from build123d import *

# Parameters (mm, degrees)
BASPROSKE_W         = 5
BASPROSKE_H         = 19
TOOTHCUT_DEPTH      = 28.331300737
TEETHCUTS_COUNT     = 17
BORSKE_R            = 4
BORE_DEPTH          = 50.0000508
BOSS_EXTRUDE1_DEPTH = 5


with BuildPart() as part:
    # BasProSke → Base-Revolve (revolve)
    with BuildSketch(Plane(origin=(0, 0, 0), x_dir=(1, 0, 0), z_dir=(0, 1, 0)), mode=Mode.PRIVATE) as base_revolve_sk:
        with Locations((2.5, 9.5)):
            Rectangle(BASPROSKE_W, BASPROSKE_H)
    revolve(base_revolve_sk.sketch.rotate(Axis((-10, 0, 0), (1, 0, 0)), 180), axis=Axis((-10, 0, 0), (1, 0, 0)))

    # TooCutSke → ToothCut (cut, through all)
    with BuildSketch(Plane(origin=(0, 0, 0), x_dir=(0, 0, -1), z_dir=(1, 0, 0))):
        with BuildLine():
            ThreePointArc((1.020352389, 14.463052306), (0, 14.499), (-1.020352389, 14.463052306))
            ThreePointArc((-1.020352389, 14.463052306), (-1.632621885, 16.804485203), (-3.026143023, 18.783192049))
            ThreePointArc((-3.026143023, 18.783192049), (0, 19.0254), (3.026143023, 18.783192049))
            ThreePointArc((3.026143023, 18.783192049), (1.632621885, 16.804485203), (1.020352389, 14.463052306))
        make_face()
    toothcut = extrude(amount=TOOTHCUT_DEPTH, mode=Mode.SUBTRACT)

    # TeethCuts: ToothCut ×17 about axis
    teethcuts_axis = Axis((0, 0, 0), (1, 0, 0))
    for i in range(1, TEETHCUTS_COUNT):
        add(toothcut.rotate(teethcuts_axis, i * 360 / TEETHCUTS_COUNT), mode=Mode.SUBTRACT)

    # BorSke → Bore (cut, symmetric)
    with BuildSketch(Plane(origin=(0, 0, 0), x_dir=(0, 0, -1), z_dir=(1, 0, 0))):
        with Locations(Location((0, 0, 0), (0, 0, 180))):
            Circle(BORSKE_R)
    extrude(amount=BORE_DEPTH, both=True, mode=Mode.SUBTRACT)

    # Sketch1 → Boss-Extrude1 (add)
    with BuildSketch(Plane(origin=(5, 0, 0), x_dir=(0, 0, -1), z_dir=(1, 0, 0))):
        with BuildLine():
            ThreePointArc((3.122498999, 2.5), (0, 4), (-3.122498999, 2.5))
            Line((-3.122498999, 2.5), (3.122498999, 2.5))
        make_face()
    extrude(amount=-BOSS_EXTRUDE1_DEPTH)


solid = part.part
Could you check a few things on this model? Use its own coordinates, in mm. A direction names the side the tool comes from. Coordinates: 2 decimals unless noted, no trailing zeros. Loops run counter-clockwise (first coordinate to the right, second up) from the corner with the lowest first, then second, coordinate; pieces in that order, holes last.
1. For faces 1 (the face through (3, 2.5, 0)), 2 (the face through (2.465, -11.386, 12.403)), 3 (the face through (2.46, 11.3, 12.48)), which set-ups out of +Z, -Z, +X, -X, +Y, -Y let a thin tool reach every point of the face, with its end or its side?
2. For P1, Ø2, axis at y = -8.5, z = -4.5, coming from the -X side; P2, Ø1.5, axis at x = 2, z = -8, coming from the -Y side; P3, Ø2, axis at x = 1, y = 6, coming from the -Z side; P4, Ø2, axis at x = 4.5, z = -4.5, coming from the -Y side, each with a flat end and sliding along its axis, tell me the tip position at first contact or that it passes through.
3. We'd pull the mould along Z, two halves only. Please class faces 4 (the face through (2.46, 16.82, -1.64)), 5 (the face through (2.54, 16.15, -10.01)), 6 (the face through (2.465, 1.352, 14.436)): released by +Z, released by -Z, zero draft, split by the parting line, or undercut.
4. Imagine slicing it at A-A (z = 0). Please give me the cut outline in (x, y), and give its area (3 significant figures).
5. I need wall thicknesses on L1, parallel to Y at x = 2.9, z = 0; L2, parallel to Y at x = 3.1, z = 16; L3, parallel to Y at x = 2.9, z = -3.5. Which ranges of each line are inside material? Lowest first, please.
Computed values:
1. face 1: +X, -X
1. face 2: +Z, +X, -X
1. face 3: +X, -X, +Y
2. P1: stops at x = 0
2. P2: stops at y = -17.56
2. P3: stops at z = -18.33
2. P4: stops at y = -17.16
3. face 4: undercut
3. face 5: released by -Z
3. face 6: released by +Z
4. outline: (0, -19) - (5, -19) - (5, -4) - (0, -4) - close; (0, 2.5) - (5, 2.5) - (5, 14.5) - (0, 14.5) - close
4. area: 135 mm2
5. L1: y = -19 to -4, 2.5 to 14.5
5. L2: y = -8.97 to -6.43, -3.1 to 0.17, 2.87 to 6.03
5. L3: y = -14.07 to -1.94, 1.94 to 18.67
